Could you check a few things on this drawing? It's one solid part, dimensions in mm from its lowest x, y, z. A direction names the side the tool comes from. Coordinates: 2 decimals unless noted, no trailing zeros. Order: outer loops, then holes, each group sorted by start corner. A loop starts at its lowest first (then second) coordinate and runs counter-clockwise, first axis right, second up. Notation, with made-up numbers: (39.5, 85) - (79.5, 85) arc R9 ccw to (79.5, 99) - close; hole circle Ø5 at (-1, 30). An arc over 180 degrees is marked (long way). Answer in a Markdown table with one row per item. Add a question column.
Item 1: If I drill on line 1 along Y through (x, z) = (11.5, 93.5); line 2 along Z through (x, y) = (35, 9); line 3 along X through (y, z) = (20.5, 7), over which ranges is the centre line in solid material (lowest first)? Write a range as from..to.
Item 2: I want a section at D-D (y = 51). Please give me the cut outline in (x, z) (1 decimal).
Item 3: I want a section at B-B (y = 6). Please give me the cut outline in (x, z) (1 decimal), plus the area to 3 significant figures.
Item 4: Thinking about a two-plate mould opening in Y: for the marked faces 3, 4, 5 and 6, which applies, +Y half, -Y half, draft (parallel to the pull), parting line (faces both ways), or undercut?
Item 5: I want a section at C-C (z = 71). Please give me the cut outline in (x, y), plus the area to 3 significant figures.
Item 6: On a 3-axis mill with a long thin cutter (end or side, diameter ignored), from which of +Z, -Z, +X, -X, +Y, -Y can I reach the whole of each face in a straight line? I mean the marked faces 1 and 2. Say none if no direction works.
Item 7: Will these pins go through, and if not, where does the flat tip stop? pin 1 Ø7 at (y, z) = (7.85, 7.18) entering from +X; pin 2 Ø6 at (x, y) = (30.5, 44) entering from -Z.
Item 8: I want a section at A-A (x = 20.5). Please give me the cut outline in (y, z).
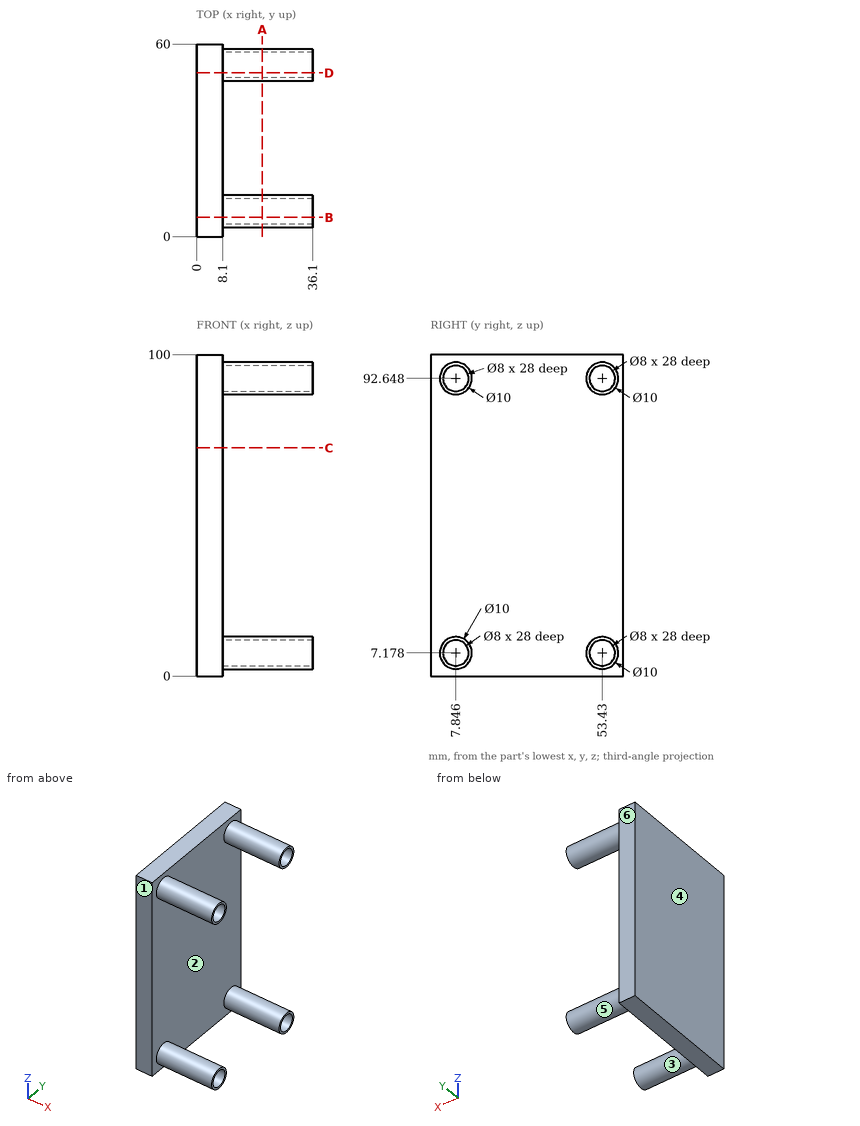
Values follow:
| question | item | result |
|---|---|---|
| 1 | line 1 | y = 2.92..3.94, 11.75..12.77, 48.5..49.52, 57.34..58.36 |
| 1 | line 2 | z = 2.31..3.35, 11.01..12.04, 87.78..88.82, 96.48..97.51 |
| 1 | line 3 | x = 0..8.1 |
| 2 | outline | (0, 0) - (8.1, 0) - (8.1, 2.8) - (36.1, 2.8) - (36.1, 4) - (8.1, 4) - (8.1, 10.4) - (36.1, 10.4) - (36.1, 11.5) - (8.1, 11.5) - (8.1, 88.3) - (36.1, 88.3) - (36.1, 89.5) - (8.1, 89.5) - (8.1, 95.8) - (36.1, 95.8) - (36.1, 97) - (8.1, 97) - (8.1, 100) - (0, 100) - close |
| 3 | outline | (0, 0) - (8.1, 0) - (8.1, 2.5) - (36.1, 2.5) - (36.1, 3.6) - (8.1, 3.6) - (8.1, 10.7) - (36.1, 10.7) - (36.1, 11.8) - (8.1, 11.8) - (8.1, 88) - (36.1, 88) - (36.1, 89.1) - (8.1, 89.1) - (8.1, 96.2) - (36.1, 96.2) - (36.1, 97.3) - (8.1, 97.3) - (8.1, 100) - (0, 100) - close |
| 3 | area | 933 mm^2 |
| 4 | face 3 | undercut |
| 4 | face 4 | draft |
| 4 | face 5 | undercut |
| 4 | face 6 | +Y half |
| 5 | outline | (0, 0) - (8.1, 0) - (8.1, 60) - (0, 60) - close |
| 5 | area | 486 mm^2 |
| 6 | face 1 | +Z, -Z, +X, -X, -Y |
| 6 | face 2 | +X |
| 7 | pin 1 | stops at x = 8.1 |
| 7 | pin 2 | passes through |
| 8 | outline | circle Ø10 at (7.85, 7.18); circle Ø10 at (7.85, 92.65); circle Ø10 at (53.43, 7.18); circle Ø10 at (53.43, 92.65); hole circle Ø8 at (7.85, 7.18); hole circle Ø8 at (7.85, 92.65); hole circle Ø8 at (53.43, 7.18); hole circle Ø8 at (53.43, 92.65) |
